```python
from build123d import *

# Parameters (mm, degrees)
SKETCH1_W             = 25
SKETCH1_H             = 15
BOSS_EXTRUDE1_DEPTH   = 3
M4X0_7_TAPPED_HOLE1_D = 3.3
CHAMFER1_SIZE         = 3


with BuildPart() as part:
    # Sketch1 → Boss-Extrude1 (new body)
    with BuildSketch(Plane(origin=(0, 0, 0), x_dir=(1, 0, 0), z_dir=(0, 1, 0))):
        Rectangle(SKETCH1_W, SKETCH1_H)
    extrude(amount=BOSS_EXTRUDE1_DEPTH)

    # M4x0.7 Tapped Hole1 (through all)
    with Locations(Plane(origin=(0, 3, 0), x_dir=(1, 0, 0), z_dir=(0, 1, 0))):
        with Locations((-7.5, 0), (7.5, 0)):
            Hole(M4X0_7_TAPPED_HOLE1_D / 2)

    # Chamfer1
    chamfer1_edges = [part.edges().sort_by_distance(p)[0] for p in [
        (0, 3, -7.5),
    ]]
    chamfer(chamfer1_edges, length=CHAMFER1_SIZE - 0.0001)  # a hair under: the kernel refuses the full size


solid = part.part
```
Check sheet for the modelled part. Datum: model origin and axes. Units: mm. Give positions to 0.01 mm unless a question says otherwise; leave off trailing zeros. Order: outer loops, then holes, each group sorted by start corner. A loop starts at its lowest first (then second) coordinate and runs counter-clockwise, first axis right, second up. Notation, with made-up numbers: (33.5, 31.25) -> (65.5, 31.25) arc R6 ccw to (65.5, 39.25) -> close; hole circle Ø10 at (-22, 76.5). An arc over 180 degrees is marked (long way). Use CSV: the item, a comma, the result in double quotes. Start each with the question number.
1) Mould release check, pull along X, two halves, no side actions. Record for faces 1 (the face through (12.5, 1, 0)), 2 (the face through (-0.2, 1.5, -6)), 3 (the face through (-5.85, 1.48, -0.07)), 4 (the face through (9.15, 1.48, -0.07)): released by +X, released by -X, zero draft, split by the parting line, or undercut.
2) Sectioned sample at A-A, the plane z = 0. Record the boundary of the cut face in (x, y), plus the area to 3 significant figures.
3) Material ranges on line 1 (X direction, y = 1, z = -0.75); line 2 (Z direction, x = -7.5, y = 1.45); line 3 (X direction, y = 2.1, z = -0.5), recorded low to high. Write a range as from..to.
4) Sectioned sample at C-C, the plane y = 2. Record the boundary of the cut face in (x, z).
5) Go/stop test with a flat-tipped pin: P1, Ø3, axis at x = 7.5, z = 0, coming from the -Y side. Record where the tip stops, or that it passes through.
Recorded:
1,face 1,"released by +X"
1,face 2,"zero draft"
1,face 3,"undercut"
1,face 4,"undercut"
2,outline,"(-12.5, 0) -> (-9.15, 0) -> (-9.15, 3) -> (-12.5, 3) -> close; (-5.85, 0) -> (5.85, 0) -> (5.85, 3) -> (-5.85, 3) -> close; (9.15, 0) -> (12.5, 0) -> (12.5, 3) -> (9.15, 3) -> close"
2,area,"55.2 mm2"
3,line 1,"-12.5..-8.97, -6.03..6.03, 8.97..12.5"
3,line 2,"-6.05..-1.65, 1.65..7.5"
3,line 3,"-12.5..-9.07, -5.93..5.93, 9.07..12.5"
4,outline,"(-12.5, -5.5) -> (12.5, -5.5) -> (12.5, 7.5) -> (-12.5, 7.5) -> close; hole circle Ø3.3 at (-7.5, 0); hole circle Ø3.3 at (7.5, 0)"
5,P1,"through"
